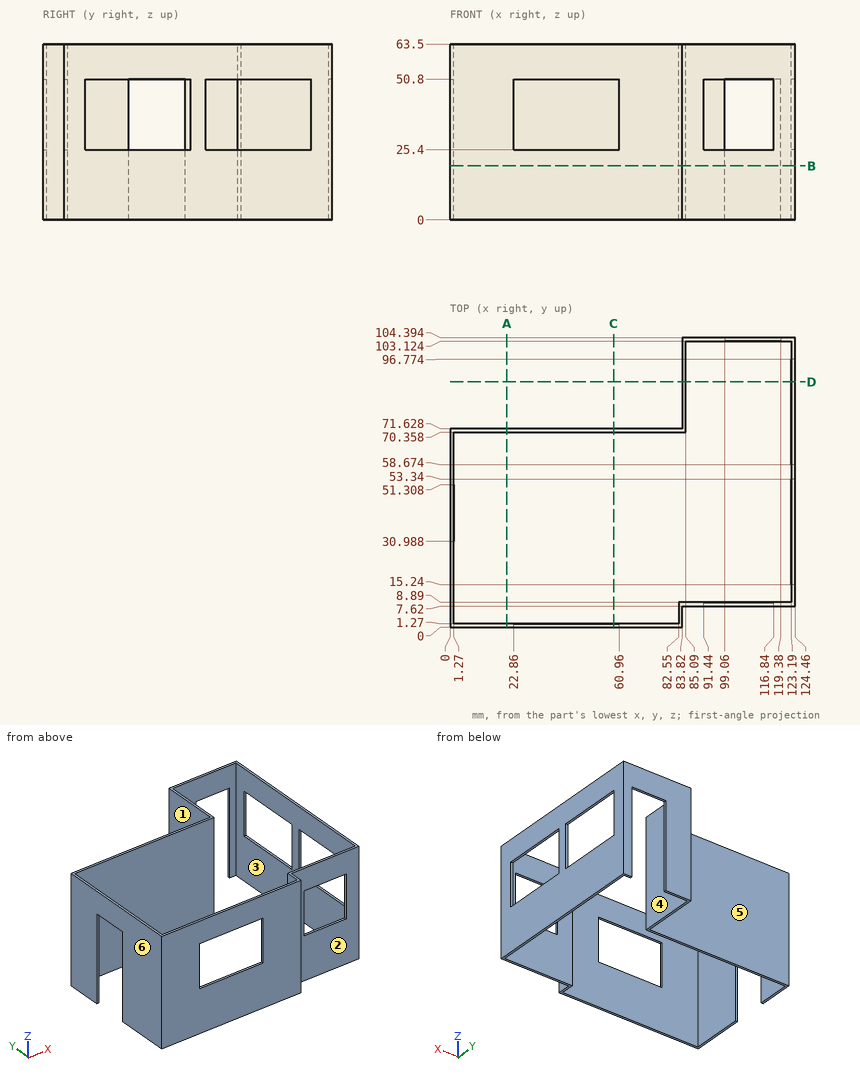
Here's the drawing with two shaded views (mm, measured from the low corner). I have some questions. A direction names the side the tool comes from. Coordinates: 2 decimals unless noted, no trailing zeros. Loops run counter-clockwise (first coordinate to the right, second up) from the corner with the lowest first, then second, coordinate; pieces in that order, holes last. Notation, with made-up numbers: M -7,68.25 L -3,68.25 A23 ccw -3,76.25 Z; hole C -34,-36.5 d11. An arc over 180 degrees is marked long. Answer as CSV lines item,"result". Start each with the question number.
1. Suppose I cut it at D-D, the plane y = 88.5. List the corners of the cut face in (x, z) for me, plus the area to 3 significant figures.
2. For the marked faces 1, 2 and 3, which set-ups out of +Z, -Z, +X, -X, +Y, -Y let a thin tool reach every point of the face, with its end or its side?
3. Thinking about a two-plate mould opening in Y: for the marked faces 4, 5 and 6, which applies, +Y half, -Y half, draft (parallel to the pull), parting line (faces both ways), or undercut?
4. Suppose I cut it at A-A, the plane x = 20.5. List the corners of the cut face in (y, z) for me.
5. Suppose I cut it at C-C, the plane x = 59. List the corners of the cut face in (y, z) for me.
6. Suppose I cut it at B-B, the plane z = 19.5. List the corners of the cut face in (x, y) for me, plus the area to 3 significant figures.
7. For pin 1 Ø12 at (x, z) = (52, 49.5) entering from -Y; pin 2 Ø6 at (y, z) = (2.5, 28) entering from +X; pin 3 Ø4 at (y, z) = (88, 32) entering from -X; pin 4 Ø6 at (x, z) = (61.5, 35.5) entering from +Y, each with a flat end and sliding along its axis, tell me the tip position at first contact or that it passes through.
8. If I drill on probe 1 along Y at (x, z) = (66, 28); probe 2 along X at (y, z) = (85.5, 23); probe 3 along Y at (x, z) = (85, 23), over which ranges is the centre line in solid material (lowest first)? Write a range as [from, to].
Output:
1,outline,"M 83.82,0 L 85.09,0 L 85.09,63.5 L 83.82,63.5 Z; M 123.19,0 L 124.46,0 L 124.46,25.4 L 123.19,25.4 Z; M 123.19,50.8 L 124.46,50.8 L 124.46,63.5 L 123.19,63.5 Z"
1,area,"129 mm^2"
2,face 1,"+Z, -Z, -X, +Y"
2,face 2,"+Z, -Z, +X, -Y"
2,face 3,"+Z, -Z"
3,face 4,"undercut"
3,face 5,"+Y half"
3,face 6,"draft"
4,outline,"M 0,0 L 1.27,0 L 1.27,63.5 L 0,63.5 Z; M 70.36,0 L 71.63,0 L 71.63,63.5 L 70.36,63.5 Z"
5,outline,"M 0,0 L 1.27,0 L 1.27,25.4 L 0,25.4 Z; M 0,50.8 L 1.27,50.8 L 1.27,63.5 L 0,63.5 Z; M 70.36,0 L 71.63,0 L 71.63,63.5 L 70.36,63.5 Z"
6,outline,"M 0,0 L 83.82,0 L 83.82,7.62 L 124.46,7.62 L 124.46,104.39 L 119.38,104.39 L 119.38,103.12 L 123.19,103.12 L 123.19,8.89 L 82.55,8.89 L 82.55,1.27 L 1.27,1.27 L 1.27,30.99 L 0,30.99 Z; M 0,51.31 L 1.27,51.31 L 1.27,70.36 L 85.09,70.36 L 85.09,103.12 L 99.06,103.12 L 99.06,104.39 L 83.82,104.39 L 83.82,71.63 L 0,71.63 Z"
6,area,"523 mm^2"
7,pin 1,"stops at y = 0"
7,pin 2,"stops at x = 83.82"
7,pin 3,"stops at x = 83.82"
7,pin 4,"stops at y = 71.63"
8,probe 1,"y = [0, 1.27], [70.36, 71.63]"
8,probe 2,"x = [83.82, 85.09], [123.19, 124.46]"
8,probe 3,"y = [7.62, 8.89], [70.36, 104.39]"
